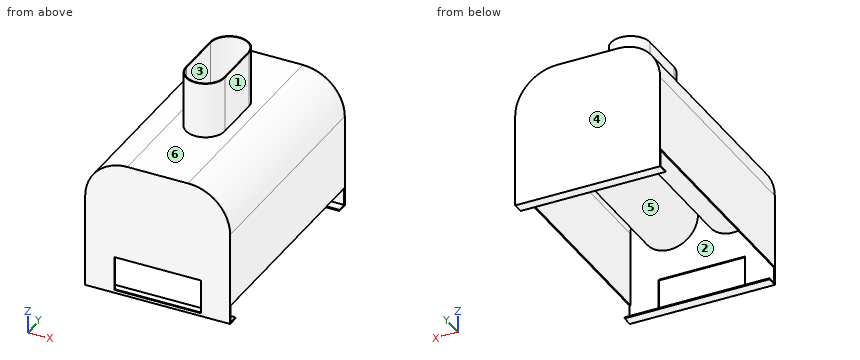
from build123d import *

# Parameters (mm, degrees)
F0_W      = 98.425
F0_H      = 92.075
F0_W_2    = 58.7375
F0_H_2    = 23.368
F1_DEPTH  = 0.79375
F2_R      = 28.575
F3_R      = 19.05
F3_R_2    = 18.25625
F4_DEPTH  = 150.8125
F5_W      = 98.425
F5_H      = 92.075
F6_DEPTH  = 0.79375
F7_R      = 28.575
F8_W      = 98.425
F8_H      = 0.79375
F9_DEPTH  = 6.35
F10_W     = 98.425
F10_H     = 0.79375
F11_DEPTH = 6.35
F13_DEPTH = 151.5745
F15_DEPTH = 2.54
F17_DEPTH = 38.1


with BuildPart() as f1:
    # F0 (on Front) → F1 (new body)
    with BuildSketch(Plane.XZ):
        with Locations((49.2125, 46.0375)):
            Rectangle(F0_W, F0_H)
        with Locations((49.2125, 13.716)):
            Rectangle(F0_W_2, F0_H_2, mode=Mode.SUBTRACT)
    extrude(amount=F1_DEPTH)

    # F2
    f2_edges = [f1.edges().sort_by_distance(p)[0] for p in [
        (0, -0.396875, 92.075),
        (98.425, -0.396875, 92.075),
    ]]
    fillet(f2_edges, radius=F2_R)

    # F3 (on face) → F4 (join)
    with BuildSketch(Plane(origin=(0, 0, 0), x_dir=(-1, 0, 0), z_dir=(0, 1, 0))):
        with Locations((-70.866, 63.754)):
            Circle(F3_R)
        with Locations((-70.866, 63.754)):
            Circle(F3_R_2, mode=Mode.SUBTRACT)
        with Locations((-27.94, 63.754)):
            Circle(F3_R)
        with Locations((-27.94, 63.754)):
            Circle(F3_R_2, mode=Mode.SUBTRACT)
    extrude(amount=F4_DEPTH)

    # F5 (on face) → F6 (join)
    with BuildSketch(Plane(origin=(0, 150.8125, 0), x_dir=(-1, 0, 0), z_dir=(0, 1, 0))):
        with Locations((-49.2125, 46.0375)):
            Rectangle(F5_W, F5_H)
    extrude(amount=F6_DEPTH)

    # F7
    f7_edges = [f1.edges().sort_by_distance(p)[0] for p in [
        (0, 151.209375, 92.075),
        (98.425, 151.209375, 92.075),
    ]]
    fillet(f7_edges, radius=F7_R)

    # F8 (on face) → F9 (join)
    with BuildSketch(Plane(origin=(0, 0, 0), x_dir=(-1, 0, 0), z_dir=(0, 1, 0))):
        with Locations((-49.2125, 0.396875)):
            Rectangle(F8_W, F8_H)
    extrude(amount=F9_DEPTH)

    # F10 (on face) → F11 (join)
    with BuildSketch(Plane.XZ.offset(-150.8125)):
        with Locations((49.2125, 0.396875)):
            Rectangle(F10_W, F10_H)
    extrude(amount=F11_DEPTH)

    # F12 (on face) → F13 (join)
    with BuildSketch(Plane(origin=(0, 0, 0), x_dir=(-1, 0, 0), z_dir=(0, 1, 0))):
        with BuildLine():
            Line((-98.425, 63.5), (-98.425, 12.7))
            Line((-98.425, 12.7), (-97.63125, 12.7))
            Line((-97.63125, 12.7), (-97.63125, 56.811744))
            ThreePointArc((-97.63125, 56.811744), (-98.225869, 60.132404), (-98.425, 63.5))
        make_face()
        with BuildLine():
            ThreePointArc((-69.85, 92.075), (-90.055576, 83.705576), (-98.425, 63.5))
            ThreePointArc((-98.425, 63.5), (-98.225869, 60.132404), (-97.63125, 56.811744))
            Line((-97.63125, 56.811744), (-97.63125, 63.5))
            ThreePointArc((-97.63125, 63.5), (-89.49431, 83.14431), (-69.85, 91.28125))
            Line((-69.85, 91.28125), (-28.575, 91.28125))
            ThreePointArc((-28.575, 91.28125), (-8.93069, 83.14431), (-0.79375, 63.5))
            Line((-0.79375, 63.5), (-0.79375, 12.7))
            Line((-0.79375, 12.7), (0, 12.7))
            Line((0, 12.7), (0, 63.5))
            ThreePointArc((0, 63.5), (-8.369424, 83.705576), (-28.575, 92.075))
            Line((-28.575, 92.075), (-69.85, 92.075))
        make_face()
    extrude(amount=F13_DEPTH)

    # F14 (on face) → F15 (cut)
    with BuildSketch(Plane.XY.offset(92.075)):
        with BuildLine():
            Line((61.9125, 62.70625), (61.9125, 94.45625))
            ThreePointArc((61.9125, 94.45625), (49.2125, 107.15625), (36.5125, 94.45625))
            Line((36.5125, 94.45625), (36.5125, 62.70625))
            ThreePointArc((36.5125, 62.70625), (49.2125, 50.00625), (61.9125, 62.70625))
        make_face()
    extrude(amount=-F15_DEPTH, mode=Mode.SUBTRACT)

    # F16 (on face) → F17 (join)
    with BuildSketch(Plane.XY.offset(92.075)):
        with BuildLine():
            Line((35.9537, 94.45625), (35.9537, 62.70625))
            ThreePointArc((35.9537, 62.70625), (49.2125, 49.44745), (62.4713, 62.70625))
            Line((62.4713, 62.70625), (62.4713, 94.45625))
            ThreePointArc((62.4713, 94.45625), (49.2125, 107.71505), (35.9537, 94.45625))
        make_face()
        with BuildLine():
            ThreePointArc((36.5125, 94.45625), (49.2125, 107.15625), (61.9125, 94.45625))
            Line((61.9125, 94.45625), (61.9125, 62.70625))
            ThreePointArc((61.9125, 62.70625), (49.2125, 50.00625), (36.5125, 62.70625))
            Line((36.5125, 62.70625), (36.5125, 94.45625))
        make_face(mode=Mode.SUBTRACT)
    extrude(amount=F17_DEPTH)


solid = f1.part
Input: part model. Units: mm. Frame: model coordinates. Face numbers are marked on the shaded views. A direction names the side the tool comes from. Coordinates: 2 decimals unless noted, no trailing zeros. Order: outer loops, then holes, each group sorted by start corner. A loop starts at its lowest first (then second) coordinate and runs counter-clockwise, first axis right, second up.
1. Cut plane B-B, the plane x = 23.5. Return loops of the section in (y, z), plus the area to 3 significant figures.
Checked values:
outline: (-0.79, 0) - (6.35, 0) - (6.35, 0.79) - (0, 0.79) - (0, 2.03) - (-0.79, 2.03) - close; (-0.79, 25.4) - (0, 25.4) - (0, 45.23) - (150.81, 45.23) - (150.81, 0.79) - (144.46, 0.79) - (144.46, 0) - (151.61, 0) - (151.61, 91.62) - (-0.79, 91.62) - close; hole (0, 46.05) - (150.81, 46.05) - (150.81, 81.46) - (0, 81.46) - close; hole (0, 82.28) - (150.81, 82.28) - (150.81, 90.81) - (0, 90.81) - close
area: 505 mm2
2. Draft query along Z for the marked faces 4, 5 and 6. Return one class per face: +Z half, -Z half, draft (parallel to the pull), parting line (faces both ways), or undercut.
Checked values:
face 4: draft
face 5: undercut
face 6: +Z half
3. Ray query, line 1 along X through (y, z) = (133, 64.5) (1 decimal); line 2 along X through (y, z) = (92, 43.5) (3 decimals); line 3 along Z through (x, y) = (81, 106.5). Return the intervals inside material, ascending.
Checked values:
line 1: x = 0 to 0.8, 8.9 to 9.7, 46.2 to 47, 51.8 to 52.6, 89.1 to 89.9, 97.6 to 98.4
line 2: x = 0 to 0.794, 97.631 to 98.425
line 3: z = 47.62 to 48.57, 78.94 to 79.88, 88.95 to 89.81
4. Cut plane A-A, the plane y = 88. Count the separate pieces of the cut face and the enclosed holes in it, plus the area to 3 significant figures.
Checked values:
separate pieces: 4
enclosed holes: 2
area: 392 mm2
5. Contact query for flat-ended pins moving along their axis: P1, Ø5, axis at x = 27, y = 3.5, coming from the +Z side (3 decimals); P2, Ø4, axis at x = 87, y = 19.5, coming from the +Z side; P3, Ø0.6, axis at x = 0.5, y = 101, coming from the -Z side. Output: stop coordinate, or through.
Checked values:
P1: stops at z = 92.075
P2: stops at z = 87.73
P3: stops at z = 12.7
6. Access query for the marked faces 1, 2 and 3. Directions: +Z, -Z, +X, -X, +Y, -Y. A direction counts if a zero-diameter tool reaches every point of the face in a straight line with its end or side. Return the directions, or none.
Checked values:
face 1: +Z, +X, +Y, -Y
face 2: none
face 3: +Z
